```python
from build123d import *

# Parameters (mm, degrees)
F1_DEPTH  = 50
F2_T      = 3
F4_DEPTH  = 50
F5_W      = 25
F5_H      = 3.5
F6_DEPTH  = 3
F7_W      = 25
F7_H      = 3.5
F8_DEPTH  = 3
F9_R      = 2
F10_R     = 1.5
F11_DEPTH = 50
F12_W     = 25
F12_H     = 3.5
F13_DEPTH = 10
F14_R     = 2


# Not quite as in the source:
# - a shell that OpenCascade refuses in one call is made with other operations: the cavity is built on its own and cut out


with BuildPart() as f1:
    # F0 (on Right) → F1 (new body)
    with BuildSketch(Plane.YZ):
        with BuildLine():
            Line((-2.5980762114, 57.9554029985), (-54.0879656003, -31.2277014993))
            Line((-54.0879656003, -31.2277014993), (48.8918131776, -31.2277014993))
            ThreePointArc((48.8918131776, -31.2277014993), (51.4898893889, -29.7277014993), (51.4898893889, -26.7277014993))
            Line((51.4898893889, -26.7277014993), (2.5980762114, 57.9554029985))
            ThreePointArc((2.5980762114, 57.9554029985), (0, 59.4554029985), (-2.5980762114, 57.9554029985))
        make_face()
    extrude(amount=F1_DEPTH)

    # F2: shell of thickness 3, made by hand


with BuildPart() as f2_core1:
    # F2_t2: copy of F1
    add(f1.part)

    # the walls: a layer under each face that stays
    f2_faces = [f2_core1.faces().sort_by_distance(p)[0] for p in [
        (25, -28.3430209058, 13.3638507496),
        (25, -2.5980762114, -31.2277014993),
        (25, 27.0439828001, 15.6138507496),
    ]]
    thicken(f2_faces, amount=-F2_T, mode=Mode.SUBTRACT)


with BuildPart() as f1_1:
    add(f1.part)

    # what is left inside the walls is the cavity
    f2_cavity = [f2_core1.part.solids().sort_by_distance(p)[0] for p in [
        (33.333333, -24.419926, 14.098851),
    ]]
    add(f2_cavity, mode=Mode.SUBTRACT)

    # F3 (on Right) → F4 (join)
    with BuildSketch(Plane.YZ):
        with BuildLine():
            Line((-54.0879656003, -31.2277014993), (-51.5879656003, -26.8975744803))
            Line((-51.5879656003, -26.8975744803), (-63.7123212533, -19.8975744803))
            Line((-63.7123212533, -19.8975744803), (-61.1142450419, -15.3975744803))
            Line((-61.1142450419, -15.3975744803), (-62.8462958495, -14.3975744803))
            ThreePointArc((-62.8462958495, -14.3975744803), (-63.6051148946, -14.2976740578), (-64.2123212533, -14.7635998841))
            Line((-64.2123212533, -14.7635998841), (-71.1197985414, -26.7277014993))
            ThreePointArc((-71.1197985414, -26.7277014993), (-71.1197985414, -29.7277014993), (-68.52172233, -31.2277014993))
            Line((-68.52172233, -31.2277014993), (-54.0879656003, -31.2277014993))
        make_face()
    extrude(amount=F4_DEPTH)

    # F5 (on face) → F6 (cut, through all)
    with BuildSketch(Plane(origin=(0, -27.0439828002, 15.6138507496), x_dir=(1, 0, 0), z_dir=(0, -0.8660254038, 0.5))):
        with Locations((37.5, -32.3379656003)):
            Rectangle(F5_W, F5_H)
    extrude(amount=-F6_DEPTH, mode=Mode.SUBTRACT)

    # F7 (on face) → F8 (cut, through all)
    with BuildSketch(Plane(origin=(0, -27.0439828002, 15.6138507496), x_dir=(1, 0, 0), z_dir=(0, -0.8660254038, 0.5))):
        with Locations((37.5, -13.8379656003)):
            Rectangle(F7_W, F7_H)
    extrude(amount=-F8_DEPTH, mode=Mode.SUBTRACT)

    # F9
    f9_edges = [f1_1.edges().sort_by_distance(p)[0] for p in [
        (50, -31.788927, 4.395365),
        (50, -33.538927, 1.364277),
        (50, -41.038927, -11.626105),
        (50, -42.788927, -14.657193),
    ]]
    fillet(f9_edges, radius=F9_R)

    # F10 (on Right) → F11 (join)
    with BuildSketch(Plane.YZ):
        with Locations((-35.9918131776, -5.8842460816)):
            Circle(F10_R)
    extrude(amount=F11_DEPTH)

    # F12 (on face) → F13 (cut)
    with BuildSketch(Plane(origin=(0, 27.0439828001, 15.6138507496), x_dir=(-1, 0, 0), z_dir=(0, 0.8660254038, 0.5))):
        with Locations((-37.5, -1.75)):
            Rectangle(F12_W, F12_H)
    extrude(amount=-F13_DEPTH, mode=Mode.SUBTRACT)

    # F14
    f14_edges = [f1_1.edges().sort_by_distance(p)[0] for p in [
        (50, 27.494945, 11.832762),
        (50, 25.744945, 14.863851),
    ]]
    fillet(f14_edges, radius=F14_R)


solid = f1_1.part
```
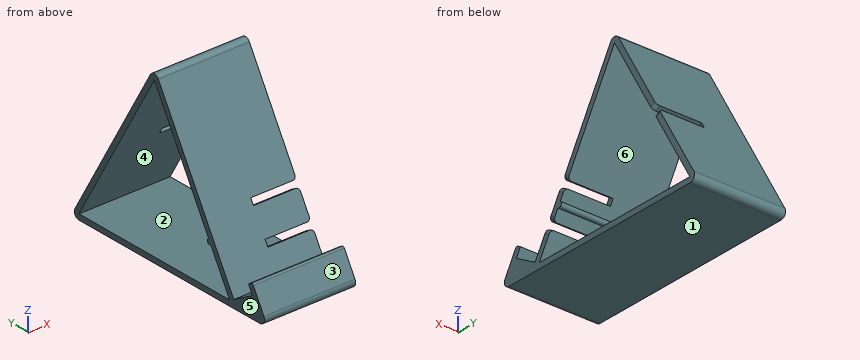
Design review of the part built by this model. Coordinates are the model's own, in mm. Face numbers are marked on the shaded views. A direction names the side the tool comes from. Round coordinates to 2 decimals unless told otherwise and drop trailing zeros. Write each loop counter-clockwise with the first axis right and the second up, starting at its lowest first coordinate (ties: lowest second). Pieces come first, ordered by that corner, then holes.
Item 1: The part is to be moulded in two halves that separate along Z. For the marked faces 3, 4, 5 and 6, say which applies: +Z half, -Z half, draft (parallel to the pull), parting line (faces both ways), or undercut.
Item 2: We need section A-A on x = 43. Write out the cut boundary in (y, z).
Item 3: For the marked faces 1 and 2, list the 3-axis set-ups (+Z, -Z, +X, -X, +Y, -Y) from which the entire face can be reached by the end or side of a thin tool; tool diameter is ignored.
Item 4: Clearance check with flat-ended pins moving along their axes: pin 1 Ø1 at (x, z) = (35.5, -12.5) entering from +Y; pin 2 Ø12 at (x, z) = (31, 0) entering from +Y; pin 3 Ø3.5 at (y, z) = (-33, 3.5) entering from +X. State where each tip first meets the part, or that it passes through.
Item 5: We need section B-B on y = 44. Write out the cut boundary in (x, z), and give its area (3 significant figures).
Item 6: For probe 1 along Y at (x, z) = (22, -16); probe 2 along Y at (x, z) = (40, -20); probe 3 along Z at (x, y) = (47, -9.5), list the stretches that pass through material, from the lowest coordinate up.
Item 7: We need section C-C on z = -23. Write out the cut boundary in (x, y).
Item 8: We need section D-D on x = 19.5. Write out the cut boundary in (y, z), and give its area (3 significant figures).
Returned:
1. face 3: +Z half
1. face 4: undercut
1. face 5: draft
1. face 6: undercut
2. outline: (-71.12, -26.73) arc R3 ccw to (-68.52, -31.23) - (48.89, -31.23) arc R3 ccw to (51.49, -26.73) - (28.79, 12.58) - (26.2, 11.08) - (48.89, -28.23) - (-48.89, -28.23) - (-41.49, -15.41) - (-44.09, -13.91) - (-51.59, -26.9) - (-63.71, -19.9) - (-61.11, -15.4) - (-62.85, -14.4) arc R1 ccw to (-64.21, -14.76) - close; (-42.34, -10.88) - (-39.74, -12.38) - (-36.74, -7.18) arc R1.5 ccw to (-35.24, -4.59) - (-32.24, 0.61) - (-34.84, 2.11) - close; (-33.09, 5.15) - (-30.49, 3.65) - (0, 56.46) - (24.45, 14.11) - (27.04, 15.61) - (2.6, 57.96) arc R3 ccw to (-2.6, 57.96) - close
3. face 1: -Z, +X, -X, +Y, -Y
3. face 2: +X, -X
4. pin 1: stops at y = 43.56
4. pin 2: stops at y = 39.52
4. pin 3: stops at x = 49.16
5. outline: (0, -31.23) - (50, -31.23) - (50, -28.23) - (0, -28.23) - close; (0, -19.75) - (50, -19.75) - (50, -13.75) - (0, -13.75) - close
5. area: 450 mm2
6. probe 1: y = -64.93 to -61.46, -45.3 to -41.83, 41.83 to 45.3
6. probe 2: y = -67.24 to -63.53, -47.61 to -44.14, 44.14 to 47.61
6. probe 3: z = -31.23 to -28.23, 40 to 46
7. outline: (0, -68.97) - (50, -68.97) - (50, -58.34) - (0, -58.34) - close; (0, -49.34) - (50, -49.34) - (50, -45.87) - (0, -45.87) - close; (0, 45.87) - (50, 45.87) - (50, 49.34) - (0, 49.34) - close
8. outline: (-71.12, -26.73) arc R3 ccw to (-68.52, -31.23) - (48.89, -31.23) arc R3 ccw to (51.49, -26.73) - (2.6, 57.96) arc R3 ccw to (-2.6, 57.96) - (-51.59, -26.9) - (-63.71, -19.9) - (-61.11, -15.4) - (-62.85, -14.4) arc R1 ccw to (-64.21, -14.76) - close; hole (-48.89, -28.23) - (48.89, -28.23) - (0, 56.46) - (-35.24, -4.59) arc R1.5 cw to (-36.74, -7.18) - close
8. area: 1,100 mm2
